Check sheet for the drawn part. Datum: minimum x, y, z corner. Units: mm. A direction names the side the tool comes from. Coordinates: 2 decimals unless noted, no trailing zeros. Loops run counter-clockwise (first coordinate to the right, second up) from the corner with the lowest first, then second, coordinate; pieces in that order, holes last. Notation, with made-up numbers: (73, 70.5) - (101, 70.5) arc R21 cw to (101, 85.5) - close; hole circle Ø5 at (68, 54.5). An arc over 180 degrees is marked (long way). Answer as CSV lines item,"result". Start each with the question number.
1. Set-up check for the marked faces 1, 2, 3, 4 and 5: record each of +Z, -Z, +X, -X, +Y, -Y from which the full face is reachable in a straight line by a thin tool's end or side.
2. Cross-section at C-C (z = 3). Enter the section's corners in (x, y).
3. Material ranges on line 1 (Y direction, x = 2.35, z = 3.75); line 2 (Y direction, x = 0.5, z = 26.5); line 3 (X direction, y = 1, z = 8.5), recorded low to high. Write a range as [from, to].
4. Gauge pin test, flat ends, axial feed: P1, Ø2.5, axis at x = 2.5, z = 22.5, coming from the +Y side; P2, Ø1.5, axis at x = 4.5, z = 7.5, coming from the +Y side; P3, Ø1.3, axis at y = 2.5, z = 1.5, coming from the +X side. Record the tip position at first contact, or that the pin passes through.
5. Cross-section at D-D (x = 1.45). Enter the section's corners in (y, z).
6. Cross-section at B-B (x = 2.5). Enter the section's corners in (y, z).
7. Cross-section at A-A (y = 3.2). Enter the section's corners in (x, z).
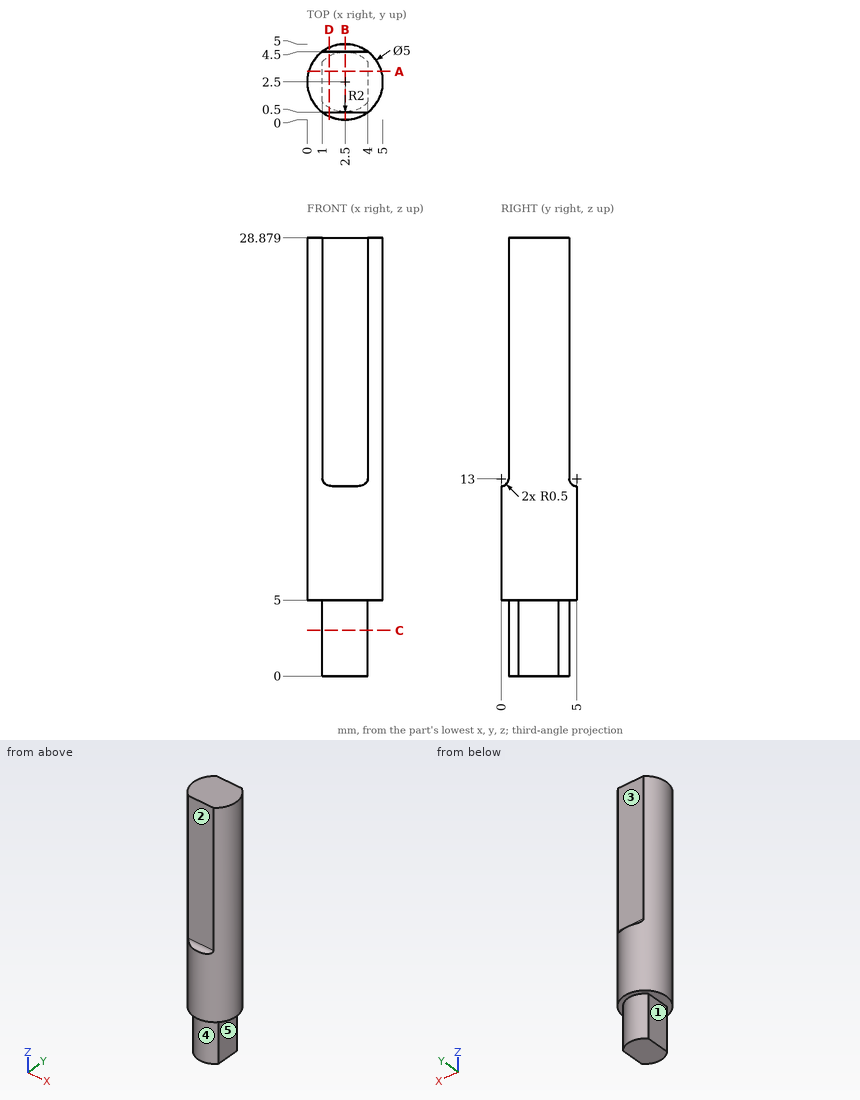
Values follow:
1,face 1,"-Z, -X, +Y, -Y"
1,face 2,"+Z, +X, -X, -Y"
1,face 3,"+Z, +X, -X, +Y"
1,face 4,"-Z, -Y"
1,face 5,"-Z, +X, +Y, -Y"
2,outline,"(1, 1.18) arc R2 ccw to (4, 1.18) - (4, 3.82) arc R2 ccw to (1, 3.82) - close"
3,line 1,"y = [0.51, 4.49]"
3,line 2,"y = [1, 4]"
3,line 3,"x = [0.5, 4.5]"
4,P1,"stops at y = 4.5"
4,P2,"stops at y = 4.67"
4,P3,"stops at x = 4"
5,outline,"(0.23, 5) - (0.8, 5) - (0.8, 0) - (4.2, 0) - (4.2, 5) - (4.77, 5) - (4.77, 12.56) arc R0.5 cw to (4.5, 13) - (4.5, 28.88) - (0.5, 28.88) - (0.5, 13) arc R0.5 cw to (0.23, 12.56) - close"
6,outline,"(0, 5) - (0.5, 5) - (0.5, 0) - (4.5, 0) - (4.5, 5) - (5, 5) - (5, 12.5) arc R0.5 cw to (4.5, 13) - (4.5, 28.88) - (0.5, 28.88) - (0.5, 13) arc R0.5 cw to (0, 12.5) - close"
7,outline,"(0.1, 5) - (1, 5) - (1, 0) - (4, 0) - (4, 5) - (4.9, 5) - (4.9, 28.88) - (0.1, 28.88) - close"
